```python
from build123d import *

# Parameters (mm, degrees)
F0_W     = 1447.8
F0_H     = 666.75
F1_DEPTH = 15.875
F2_W     = 88.9
F2_H     = 76.2
F3_DEPTH = 15.876
F4_W     = 1270
F4_H     = 76.2
F5_DEPTH = 15.876


with BuildPart() as f1:
    # F0 (on Top) → F1 (new body)
    with BuildSketch(Plane.XY):
        Rectangle(F0_W, F0_H)
    extrude(amount=F1_DEPTH)

    # F2 (on face) → F3 (cut, through all)
    with BuildSketch(Plane.XY.offset(15.875)):
        with Locations((-679.45, -295.275)):
            Rectangle(F2_W, F2_H)
        with Locations((-679.45, 295.275)):
            Rectangle(F2_W, F2_H)
        with Locations((679.45, 295.275)):
            Rectangle(F2_W, F2_H)
        with Locations((679.45, -295.275)):
            Rectangle(F2_W, F2_H)
    extrude(amount=-F3_DEPTH, mode=Mode.SUBTRACT)

    # F4 (on face) → F5 (cut, through all)
    with BuildSketch(Plane.XY.offset(15.875)):
        Polygon((-723.9, 257.175), (-723.9, 215.9), (723.9, 215.9), (723.9, 257.175), (635, 257.175), (-635, 257.175), align=None)
        with Locations((0, 295.275)):
            Rectangle(F4_W, F4_H)
    extrude(amount=-F5_DEPTH, mode=Mode.SUBTRACT)


solid = f1.part
```
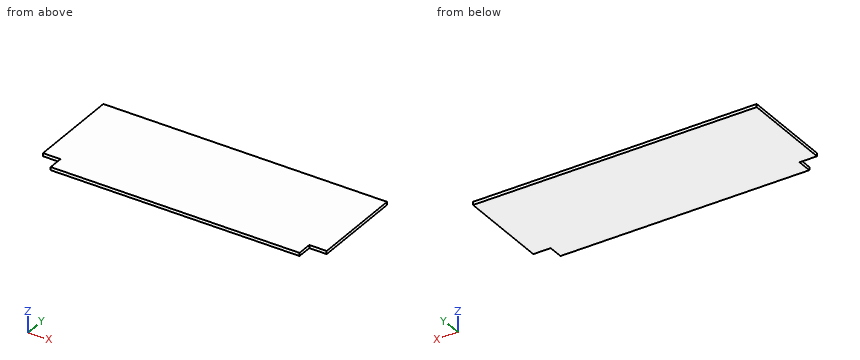
Can you work these out from the model? Positions are in its coordinate system, mm. Coordinates: 2 decimals unless noted, no trailing zeros. Write each loop counter-clockwise with the first axis right and the second up, starting at its lowest first coordinate (ties: lowest second). Pieces come first, ordered by that corner, then holes. Notation, with made-up numbers: (-12.5, -18.5) - (16.5, -18.5) arc R26 cw to (16.5, -4.5) - close; hole circle Ø2 at (-16.75, 67). An arc over 180 degrees is marked (long way). Return JSON: item names as keys, results as strings.
Q1. I'm going to push flat-ended pins straight in: pin 1 Ø5 at (y, z) = (-297.5, 4.5) entering from -X; pin 2 Ø5 at (x, z) = (686, 11) entering from -Y (3 decimals). Where does each tip first touch, or does it pass through?
Computed values:
{"pin 1": "stops at x = -635", "pin 2": "stops at y = -257.175"}
Q2. If we section it at A-A (z = 7): Please give me the cut outline in (x, y) (3 decimals).
Computed values:
{"outline": "(-723.9, -257.175) - (-635, -257.175) - (-635, -333.375) - (635, -333.375) - (635, -257.175) - (723.9, -257.175) - (723.9, 215.9) - (-723.9, 215.9) - close"}
Q3. Please list where these lines run through material, in increasing order: L1, parallel to X at y = -293, z = 7; L2, parallel to Y at x = 655.5, z = 7.5 (3 decimals). Write a range as from..to.
Computed values:
{"L1": "x = -635..635", "L2": "y = -257.175..215.9"}
